from build123d import *

# Parameters (mm, degrees)
F1_DEPTH = 160


# Not quite as in the source:
# - ends of sketch curves that miss each other by under 0.0002 mm in the source are joined
# - the program builds the solid bodies; features that only make, move or delete a surface that nothing else refers to are left out


with BuildPart() as f1:
    # F0 (on Top) → F1 (new body)
    with BuildSketch(Plane.XY):
        with BuildLine():
            Line((3.939341, -5), (6.799995, -7.860656))
            Line((6.799995, -7.860656), (6.799995, -12.199997))
            ThreePointArc((6.799995, -12.199997), (6.7121307415, -12.4121300846), (6.5, -12.5))
            Line((6.5, -12.5), (4.599998, -12.5))
            ThreePointArc((4.599998, -12.5), (4.2464446094, -12.6464466094), (4.099998, -13))
            Line((4.099998, -13), (4.099998, -14.699997))
            ThreePointArc((4.099998, -14.699997), (4.1878632585, -14.9121300846), (4.399994, -15))
            Line((4.399994, -15), (12.5, -15))
            ThreePointArc((12.5, -15), (14.267766953, -14.267766953), (15, -12.5))
            Line((15, -12.5), (15, -4.399994))
            ThreePointArc((15, -4.399994), (14.9121300846, -4.1878632585), (14.699997, -4.099999))
            Line((14.699997, -4.099999), (13, -4.099998))
            ThreePointArc((13, -4.099998), (12.6464466094, -4.2464446094), (12.5, -4.599998))
            Line((12.5, -4.599998), (12.5, -6.5))
            ThreePointArc((12.5, -6.5), (12.4121300846, -6.7121307415), (12.199997, -6.799995))
            Line((12.199997, -6.799995), (7.860655, -6.799995))
            Line((7.860655, -6.799995), (5, -3.93934))
            Line((5, -3.93934), (5, 3.939341))
            Line((5, 3.939341), (7.860655, 6.799995))
            Line((7.860655, 6.799995), (12.199997, 6.799995))
            ThreePointArc((12.199997, 6.799995), (12.4121300846, 6.7121307415), (12.5, 6.5))
            Line((12.5, 6.5), (12.5, 4.599998))
            ThreePointArc((12.5, 4.599998), (12.6464466094, 4.2464446094), (13, 4.099998))
            Line((13, 4.099998), (14.699997, 4.099998))
            ThreePointArc((14.699997, 4.099998), (14.9121300846, 4.1878632585), (15, 4.399994))
            Line((15, 4.399994), (15, 12.5))
            ThreePointArc((15, 12.5), (14.267766953, 14.267766953), (12.5, 15))
            Line((12.5, 15), (4.399994, 15))
            ThreePointArc((4.399994, 15), (4.1878632585, 14.9121300846), (4.099999, 14.699997))
            Line((4.099999, 14.699997), (4.099998, 13))
            ThreePointArc((4.099998, 13), (4.2464446094, 12.6464466094), (4.599998, 12.5))
            Line((4.599998, 12.5), (6.5, 12.5))
            ThreePointArc((6.5, 12.5), (6.7121307415, 12.4121300846), (6.799995, 12.199997))
            Line((6.799995, 12.199997), (6.799995, 7.860655))
            Line((6.799995, 7.860655), (3.939341, 5))
            Line((3.939341, 5), (-3.93934, 5))
            Line((-3.93934, 5), (-6.799995, 7.860655))
            Line((-6.799995, 7.860655), (-6.799995, 12.199997))
            ThreePointArc((-6.799995, 12.199997), (-6.7121307415, 12.4121300846), (-6.5, 12.5))
            Line((-6.5, 12.5), (-4.599998, 12.5))
            ThreePointArc((-4.599998, 12.5), (-4.2464446094, 12.6464466094), (-4.099998, 13))
            Line((-4.099998, 13), (-4.099998, 14.699997))
            ThreePointArc((-4.099998, 14.699997), (-4.1878632585, 14.9121300846), (-4.399994, 15))
            Line((-4.399994, 15), (-12.5, 15))
            ThreePointArc((-12.5, 15), (-14.267766953, 14.267766953), (-15, 12.5))
            Line((-15, 12.5), (-15, 4.399994))
            ThreePointArc((-15, 4.399994), (-14.9121300846, 4.1878632585), (-14.699997, 4.099999))
            Line((-14.699997, 4.099999), (-13, 4.099998))
            ThreePointArc((-13, 4.099998), (-12.6464466094, 4.2464446094), (-12.5, 4.599998))
            Line((-12.5, 4.599998), (-12.5, 6.5))
            ThreePointArc((-12.5, 6.5), (-12.4121300846, 6.7121307415), (-12.199997, 6.799995))
            Line((-12.199997, 6.799995), (-7.860656, 6.799995))
            Line((-7.860656, 6.799995), (-5, 3.939341))
            Line((-5, 3.939341), (-5, -3.93934))
            Line((-5, -3.93934), (-7.860656, -6.799995))
            Line((-7.860656, -6.799995), (-12.199997, -6.799995))
            ThreePointArc((-12.199997, -6.799995), (-12.4121300846, -6.7121307415), (-12.5, -6.5))
            Line((-12.5, -6.5), (-12.5, -4.599998))
            ThreePointArc((-12.5, -4.599998), (-12.6464466094, -4.2464446094), (-13, -4.099998))
            Line((-13, -4.099998), (-14.699997, -4.099998))
            ThreePointArc((-14.699997, -4.099998), (-14.9121300846, -4.1878632585), (-15, -4.399994))
            Line((-15, -4.399994), (-15, -12.5))
            ThreePointArc((-15, -12.5), (-14.267766953, -14.267766953), (-12.5, -15))
            Line((-12.5, -15), (-4.399994, -15))
            ThreePointArc((-4.399994, -15), (-4.1878632585, -14.9121300846), (-4.099999, -14.699997))
            Line((-4.099999, -14.699997), (-4.099998, -13))
            ThreePointArc((-4.099998, -13), (-4.2464446094, -12.6464466094), (-4.599998, -12.5))
            Line((-4.599998, -12.5), (-6.5, -12.5))
            ThreePointArc((-6.5, -12.5), (-6.7121307415, -12.4121300846), (-6.799995, -12.199997))
            Line((-6.799995, -12.199997), (-6.799995, -7.860656))
            Line((-6.799995, -7.860656), (-3.93934, -5))
            Line((-3.93934, -5), (3.939341, -5))
        make_face()
        with BuildLine():
            Line((-8.299995, -14), (-12.5, -14))
            ThreePointArc((-12.5, -14), (-13.5606601718, -13.5606601718), (-14, -12.5))
            Line((-14, -12.5), (-14, -8.299995))
            ThreePointArc((-14, -8.299995), (-13.8535533906, -7.9464416094), (-13.5, -7.799995))
            Line((-13.5, -7.799995), (-9.299995, -7.799995))
            ThreePointArc((-9.299995, -7.799995), (-8.2393348282, -8.2393348282), (-7.799995, -9.299995))
            Line((-7.799995, -9.299995), (-7.799995, -13.5))
            ThreePointArc((-7.799995, -13.5), (-7.9464416094, -13.8535533906), (-8.299995, -14))
        make_face(mode=Mode.SUBTRACT)
        with BuildLine():
            Line((12.5, -14), (8.299995, -14))
            ThreePointArc((8.299995, -14), (7.9464416094, -13.8535533906), (7.799995, -13.5))
            Line((7.799995, -13.5), (7.799995, -9.299995))
            ThreePointArc((7.799995, -9.299995), (8.2393348282, -8.2393348282), (9.299995, -7.799995))
            Line((9.299995, -7.799995), (13.5, -7.799995))
            ThreePointArc((13.5, -7.799995), (13.8535533906, -7.9464416094), (14, -8.299995))
            Line((14, -8.299995), (14, -12.5))
            ThreePointArc((14, -12.5), (13.5606601718, -13.5606601718), (12.5, -14))
        make_face(mode=Mode.SUBTRACT)
        with BuildLine():
            Line((3.657288, -2.243073), (3.878887, -3.285876))
            ThreePointArc((3.878887, -3.285876), (3.7433613906, -3.7433613906), (3.2858769836, -3.8788870773))
            Line((3.2858769836, -3.8788870773), (2.243074, -3.657287))
            Line((2.243074, -3.657287), (2.005135, -3.419348))
            ThreePointArc((2.005135, -3.419348), (1.841799908, -3.3354753308), (1.6601868142, -3.3624816237))
            ThreePointArc((1.6601868142, -3.3624816237), (0, -3.75), (-1.6601870383, -3.3624810777))
            ThreePointArc((-1.6601870383, -3.3624810777), (-1.841799908, -3.3354753308), (-2.0051340344, -3.4193479656))
            Line((-2.0051340344, -3.4193479656), (-2.243073, -3.657287))
            Line((-2.243073, -3.657287), (-3.285876, -3.878887))
            ThreePointArc((-3.285876, -3.878887), (-3.7433613906, -3.7433613906), (-3.8788870773, -3.2858769836))
            Line((-3.8788870773, -3.2858769836), (-3.657287, -2.243073))
            Line((-3.657287, -2.243073), (-3.419348, -2.005134))
            ThreePointArc((-3.419348, -2.005134), (-3.3354753308, -1.841799908), (-3.3624816237, -1.6601868142))
            ThreePointArc((-3.3624816237, -1.6601868142), (-3.75, 0), (-3.3624810777, 1.6601870383))
            ThreePointArc((-3.3624810777, 1.6601870383), (-3.3354753883, 1.8418002569), (-3.4193484656, 2.0051345344))
            Line((-3.4193484656, 2.0051345344), (-3.657287, 2.243074))
            Line((-3.657287, 2.243074), (-3.878887, 3.285877))
            ThreePointArc((-3.878887, 3.285877), (-3.7433613906, 3.7433613906), (-3.2858769836, 3.8788870773))
            Line((-3.2858769836, 3.8788870773), (-2.243073, 3.657288))
            Line((-2.243073, 3.657288), (-2.005134, 3.419348))
            ThreePointArc((-2.005134, 3.419348), (-1.8418001264, 3.3354753668), (-1.6601872112, 3.3624814277))
            ThreePointArc((-1.6601872112, 3.3624814277), (0, 3.75), (1.6601870383, 3.3624810777))
            ThreePointArc((1.6601870383, 3.3624810777), (1.8418002569, 3.3354753883), (2.0051345344, 3.4193484656))
            Line((2.0051345344, 3.4193484656), (2.243074, 3.657288))
            Line((2.243074, 3.657288), (3.285877, 3.878887))
            ThreePointArc((3.285877, 3.878887), (3.7433610448, 3.7433617364), (3.8788872806, 3.2858779404))
            Line((3.8788872806, 3.2858779404), (3.657288, 2.243074))
            Line((3.657288, 2.243074), (3.419348, 2.005135))
            ThreePointArc((3.419348, 2.005135), (3.3354753668, 1.8418001264), (3.3624814277, 1.6601872112))
            ThreePointArc((3.3624814277, 1.6601872112), (3.75, 0), (3.3624810777, -1.6601870383))
            ThreePointArc((3.3624810777, -1.6601870383), (3.3354753308, -1.841799908), (3.4193479656, -2.0051340344))
            Line((3.4193479656, -2.0051340344), (3.657288, -2.243073))
        make_face(mode=Mode.SUBTRACT)
        with BuildLine():
            Line((-9.299995, 7.799995), (-13.5, 7.799995))
            ThreePointArc((-13.5, 7.799995), (-13.8535533906, 7.9464416094), (-14, 8.299995))
            Line((-14, 8.299995), (-14, 12.5))
            ThreePointArc((-14, 12.5), (-13.5606601718, 13.5606601718), (-12.5, 14))
            Line((-12.5, 14), (-8.299995, 14))
            ThreePointArc((-8.299995, 14), (-7.9464416094, 13.8535533906), (-7.799995, 13.5))
            Line((-7.799995, 13.5), (-7.799995, 9.299995))
            ThreePointArc((-7.799995, 9.299995), (-8.2393348282, 8.2393348282), (-9.299995, 7.799995))
        make_face(mode=Mode.SUBTRACT)
        with BuildLine():
            Line((13.5, 7.799995), (9.299995, 7.799995))
            ThreePointArc((9.299995, 7.799995), (8.2393348282, 8.2393348282), (7.799995, 9.299995))
            Line((7.799995, 9.299995), (7.799995, 13.5))
            ThreePointArc((7.799995, 13.5), (7.9464416094, 13.8535533906), (8.299995, 14))
            Line((8.299995, 14), (12.5, 14))
            ThreePointArc((12.5, 14), (13.5606601718, 13.5606601718), (14, 12.5))
            Line((14, 12.5), (14, 8.299995))
            ThreePointArc((14, 8.299995), (13.8535533906, 7.9464416094), (13.5, 7.799995))
        make_face(mode=Mode.SUBTRACT)
    extrude(amount=F1_DEPTH)


solid = f1.part
Source: CAD feature listing. Evaluate the final solid. Frame: model axes, mm. A direction names the side the tool comes from. Give positions to 0.01 mm unless a question says otherwise; leave off trailing zeros. Order: outer loops, then holes, each group sorted by start corner. A loop starts at its lowest first (then second) coordinate and runs counter-clockwise, first axis right, second up. Notation, with made-up numbers: (-10.75, -12) -> (37.25, -12) arc R23 ccw to (37.25, 20) -> close; hole circle Ø5 at (-33, -37.5). An arc over 180 degrees is marked (long way). Write item = value, one per line.
Item 1: Contact query for flat-ended pins moving along their axis: pin 1 (4 mm diameter, centred on x = -9.5, y = -3, fed in from -Z); pin 2 (2.5 mm diameter, centred on x = 0, z = 42, fed in from -Y); pin 3 (1.4 mm diameter, centred on x = 13.5, z = 59, fed in from -Y). Output: stop coordinate, or through.
Check result:
pin_1 = through
pin_2 = -5
pin_3 = -14.98
Item 2: Section query A-A (y = 0). Output: boundary loops of the cut face in (x, z), then the cut area to 3 significant figures.
Check result:
outline = (-5, 0) -> (-3.75, 0) -> (-3.75, 160) -> (-5, 160) -> close; (3.75, 0) -> (5, 0) -> (5, 160) -> (3.75, 160) -> close
area = 400 mm²
Item 3: Mould query, pull axis X, two halves, no side actions, for faces 4 (the face through (14.248, -14.287, 78.88)), 5 (the face through (-10, 14, 79)), 6 (the face through (-15, 9, 79)). Classes: +X half, -X half, draft (parallel to the pull), parting line (faces both ways), or undercut.
Check result:
face_4 = +X half
face_5 = undercut
face_6 = -X half
Item 4: Ray query, probe 1 along X at (y, z) = (9, 108); probe 2 along Y at (x, z) = (9.75, 49.5); probe 3 along Y at (x, z) = (-1.5, 123). Return the intervals inside material, ascending.
Check result:
probe_1 = -15 to -14, -7.83 to -6.8, 6.8 to 7.83, 14 to 15
probe_2 = -15 to -14, -7.8 to -6.8, 6.8 to 7.8, 14 to 15
probe_3 = -5 to -3.44, 3.44 to 5
Item 5: Section query B-B (y = -10.75). Output: boundary loops of the cut face in (x, z).
Check result:
outline = (-15, 0) -> (-14, 0) -> (-14, 160) -> (-15, 160) -> close; (-7.8, 0) -> (-6.8, 0) -> (-6.8, 160) -> (-7.8, 160) -> close; (6.8, 0) -> (7.8, 0) -> (7.8, 160) -> (6.8, 160) -> close; (14, 0) -> (15, 0) -> (15, 160) -> (14, 160) -> close
Item 6: Set-up query: faces 1 (the face through (11, -7.8, 79)), 2 (the face through (0, -5, 79)), 3 (the face through (-5, 0, 79)). Return all of +Z, -Z, +X, -X, +Y, -Y with unobstructed straight access to the full face (end or side cutting, diameter ignored); none if empty.
Check result:
face_1 = +Z, -Z
face_2 = +Z, -Z, -Y
face_3 = +Z, -Z, -X
Item 7: Section query C-C (z = 25). State how many separate pieces and enclosed holes the cut face has, then the cut area to 3 significant figures.
Check result:
separate_pieces = 1
enclosed_holes = 5
area = 234 mm²
